Here's how the part is built. I have some questions about the finished solid (model axes, mm). Face numbers are marked on the shaded views. Give positions to 0.01 mm unless a question says otherwise; leave off trailing zeros. Write each loop counter-clockwise with the first axis right and the second up, starting at its lowest first coordinate (ties: lowest second). Pieces come first, ordered by that corner, then holes. Notation, with made-up numbers: (31, 26) -> (54, 26) arc R30 cw to (54, 50) -> close; hole circle Ø2 at (3.5, -25). An arc over 180 degrees is marked (long way). Put each result on its own line as item: value. Start each with the question number.
from build123d import *

# Parameters (mm, degrees)
SKETCH1_R             = 0.25
BOSS_EXTRUDE1_DEPTH   = 2.7
BOSS_EXTRUDE1_2_DEPTH = 2.7
BOSS_EXTRUDE1_3_DEPTH = 2.7
BOSS_EXTRUDE1_4_DEPTH = 2.7
BOSS_EXTRUDE1_5_DEPTH = 2.7
BOSS_EXTRUDE1_6_DEPTH = 2.7
BOSS_EXTRUDE1_7_DEPTH = 2.7
BOSS_EXTRUDE1_8_DEPTH = 2.7
SKETCH1_7_W           = 13.5
SKETCH1_7_H           = 2.85
SKETCH1_7_W_2         = 13.1
SKETCH1_7_H_2         = 2.45
BOSS_EXTRUDE3_DEPTH   = 2.7
SKETCH1_8_W           = 13.1
SKETCH1_8_H           = 2.45
SKETCH1_8_R           = 0.25
BOSS_EXTRUDE4_DEPTH   = 0.2
SKETCH1_9_R           = 0.25
BOSS_EXTRUDE5_DEPTH   = 2.7


with BuildPart() as part:
    # Sketch1 → Boss-Extrude1 (new body)
    with BuildSketch(Plane(origin=(0, 0, 0), x_dir=(1, 0, 0), z_dir=(0, 1, 0))):
        with Locations((-3.403301887, 0.02370283)):
            Circle(SKETCH1_R)
    extrude(amount=-BOSS_EXTRUDE1_DEPTH)



with BuildPart() as body_2:
    # Sketch1 → Boss-Extrude1 2 (new body)
    with BuildSketch(Plane(origin=(0, 0, 0), x_dir=(1, 0, 0), z_dir=(0, 1, 0))):
        with Locations((-1.903301887, 0.02370283)):
            Circle(SKETCH1_R)
    extrude(amount=-BOSS_EXTRUDE1_2_DEPTH)


with BuildPart() as body_3:
    # Sketch1 → Boss-Extrude1 3 (new body)
    with BuildSketch(Plane(origin=(0, 0, 0), x_dir=(1, 0, 0), z_dir=(0, 1, 0))):
        with Locations((-0.403301887, 0.02370283)):
            Circle(SKETCH1_R)
    extrude(amount=-BOSS_EXTRUDE1_3_DEPTH)


with BuildPart() as body_4:
    # Sketch1 → Boss-Extrude1 4 (new body)
    with BuildSketch(Plane(origin=(0, 0, 0), x_dir=(1, 0, 0), z_dir=(0, 1, 0))):
        with Locations((1.096698113, 0.02370283)):
            Circle(SKETCH1_R)
    extrude(amount=-BOSS_EXTRUDE1_4_DEPTH)


with BuildPart() as body_5:
    # Sketch1 → Boss-Extrude1 5 (new body)
    with BuildSketch(Plane(origin=(0, 0, 0), x_dir=(1, 0, 0), z_dir=(0, 1, 0))):
        with Locations((2.596698113, 0.02370283)):
            Circle(SKETCH1_R)
    extrude(amount=-BOSS_EXTRUDE1_5_DEPTH)


with BuildPart() as body_6:
    # Sketch1 → Boss-Extrude1 6 (new body)
    with BuildSketch(Plane(origin=(0, 0, 0), x_dir=(1, 0, 0), z_dir=(0, 1, 0))):
        with Locations((4.096698113, 0.02370283)):
            Circle(SKETCH1_R)
    extrude(amount=-BOSS_EXTRUDE1_6_DEPTH)


with BuildPart() as body_7:
    # Sketch1 → Boss-Extrude1 7 (new body)
    with BuildSketch(Plane(origin=(0, 0, 0), x_dir=(1, 0, 0), z_dir=(0, 1, 0))):
        with Locations((5.596698113, 0.02370283)):
            Circle(SKETCH1_R)
    extrude(amount=-BOSS_EXTRUDE1_7_DEPTH)


with BuildPart() as body_8:
    # Sketch1 → Boss-Extrude1 8 (new body)
    with BuildSketch(Plane(origin=(0, 0, 0), x_dir=(1, 0, 0), z_dir=(0, 1, 0))):
        with Locations((7.096698113, 0.02370283)):
            Circle(SKETCH1_R)
    extrude(amount=-BOSS_EXTRUDE1_8_DEPTH)


with BuildPart() as body_9:
    # Sketch1_7 → Boss-Extrude3 (new body)
    with BuildSketch(Plane(origin=(0, 0, 0), x_dir=(1, 0, 0), z_dir=(0, 1, 0))):
        with Locations((1.846698113, -0.098128497)):
            Rectangle(SKETCH1_7_W, SKETCH1_7_H)
        with Locations((1.846698113, -0.098128497)):
            Rectangle(SKETCH1_7_W_2, SKETCH1_7_H_2, mode=Mode.SUBTRACT)
    extrude(amount=BOSS_EXTRUDE3_DEPTH)

    # Sketch1_8 → Boss-Extrude4 (add)
    with BuildSketch(Plane(origin=(0, 0, 0), x_dir=(1, 0, 0), z_dir=(0, 1, 0))):
        with Locations((1.846698113, -0.098128497)):
            Rectangle(SKETCH1_8_W, SKETCH1_8_H)
        with Locations((-3.403301887, 0.02370283)):
            Circle(SKETCH1_8_R, mode=Mode.SUBTRACT)
        with Locations((-1.903301887, 0.02370283)):
            Circle(SKETCH1_8_R, mode=Mode.SUBTRACT)
        with Locations((-0.403301887, 0.02370283)):
            Circle(SKETCH1_8_R, mode=Mode.SUBTRACT)
        with Locations((1.096698113, 0.02370283)):
            Circle(SKETCH1_8_R, mode=Mode.SUBTRACT)
        with Locations((2.596698113, 0.02370283)):
            Circle(SKETCH1_8_R, mode=Mode.SUBTRACT)
        with Locations((4.096698113, 0.02370283)):
            Circle(SKETCH1_8_R, mode=Mode.SUBTRACT)
        with Locations((5.596698113, 0.02370283)):
            Circle(SKETCH1_8_R, mode=Mode.SUBTRACT)
        with Locations((7.096698113, 0.02370283)):
            Circle(SKETCH1_8_R, mode=Mode.SUBTRACT)
    extrude(amount=BOSS_EXTRUDE4_DEPTH)


with BuildPart() as part_1:
    add(part.part)

    add(body_2.part)  # Boss-Extrude5 merges body 2

    add(body_3.part)  # Boss-Extrude5 merges body 3

    add(body_4.part)  # Boss-Extrude5 merges body 4

    add(body_5.part)  # Boss-Extrude5 merges body 5

    add(body_6.part)  # Boss-Extrude5 merges body 6

    add(body_7.part)  # Boss-Extrude5 merges body 7

    add(body_8.part)  # Boss-Extrude5 merges body 8

    add(body_9.part)  # Boss-Extrude5 merges body 9
    # Sketch1_9 → Boss-Extrude5 (add)
    with BuildSketch(Plane(origin=(0, 0, 0), x_dir=(1, 0, 0), z_dir=(0, 1, 0))):
        with Locations((-3.403301887, 0.02370283)):
            Circle(SKETCH1_9_R)
        with Locations((-0.403301887, 0.02370283)):
            Circle(SKETCH1_9_R)
        with Locations((1.096698113, 0.02370283)):
            Circle(SKETCH1_9_R)
        with Locations((2.596698113, 0.02370283)):
            Circle(SKETCH1_9_R)
        with Locations((4.096698113, 0.02370283)):
            Circle(SKETCH1_9_R)
        with Locations((5.596698113, 0.02370283)):
            Circle(SKETCH1_9_R)
        with Locations((7.096698113, 0.02370283)):
            Circle(SKETCH1_9_R)
        with Locations((-1.903301887, 0.02370283)):
            Circle(SKETCH1_9_R)
    extrude(amount=BOSS_EXTRUDE5_DEPTH)


solid = part_1.part
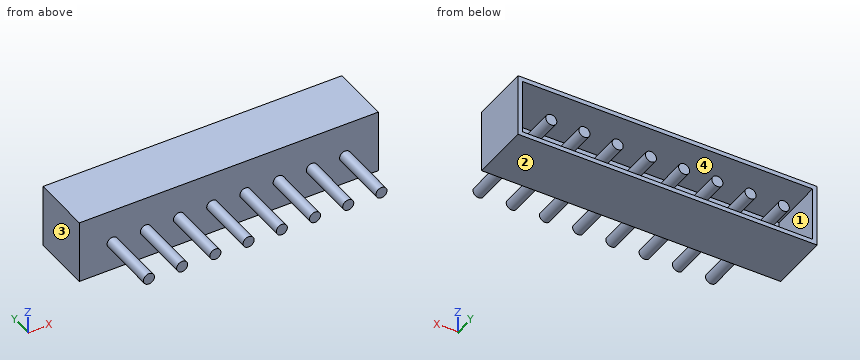
1) I want a section at A-A, the plane y = 2.05. State how many separate pieces and enclosed holes the cut face has, and give its area (3 significant figures).
2) I want a section at C-C, the plane x = -1. Write out the boundary of the cut face in (y, z).
3) I'm going to push flat-ended pins straight in: pin 1 Ø0.9 at (x, z) = (-1, -0.5) entering from -Y; pin 2 Ø1.2 at (x, z) = (3, 0) entering from +Y. Where does each tip first touch, or does it pass through?
4) I want a section at D-D, the plane y = -1.95. Write out the boundary of the cut face in (x, z), and give its area (3 significant figures).
5) I want a section at B-B, the plane z = 0.4. Write out the boundary of the cut face in (x, y), and give its area (3 significant figures).
6) Thinking about a two-plate mould opening in Z: for the marked faces 1, 2, 3 and 4, which applies, released by +Z, released by -Z, zero draft, split by the parting line, or undercut?
7) I need wall thicknesses on probe 1 along Z at (x, y) = (7.75, 0.7); probe 2 along Z at (x, y) = (-3.25, 1.8); probe 3 along Z at (x, y) = (-0.5, 2.15). Which ranges of each line are inside material? Lowest first, please.
Established:
1. separate pieces: 9
1. enclosed holes: 1
1. area: 7.95 mm2
2. outline: (0, -1.33) -> (2.7, -1.33) -> (2.7, -1.13) -> (0.2, -1.13) -> (0.2, 1.32) -> (2.7, 1.32) -> (2.7, 1.52) -> (0, 1.52) -> close
3. pin 1: stops at y = 0
3. pin 2: stops at y = 2.7
4. outline: circle Ø0.5 at (-3.4, -0.02); circle Ø0.5 at (-1.9, -0.02); circle Ø0.5 at (-0.4, -0.02); circle Ø0.5 at (1.1, -0.02); circle Ø0.5 at (2.6, -0.02); circle Ø0.5 at (4.1, -0.02); circle Ø0.5 at (5.6, -0.02); circle Ø0.5 at (7.1, -0.02)
4. area: 1.57 mm2
5. outline: (-4.9, 0) -> (8.6, 0) -> (8.6, 2.7) -> (8.4, 2.7) -> (8.4, 0.2) -> (-4.7, 0.2) -> (-4.7, 2.7) -> (-4.9, 2.7) -> close
5. area: 3.70 mm2
6. face 1: undercut
6. face 2: released by -Z
6. face 3: zero draft
6. face 4: undercut
7. probe 1: z = -1.33 to -1.13, 1.32 to 1.52
7. probe 2: z = -1.33 to -1.13, -0.22 to 0.17, 1.32 to 1.52
7. probe 3: z = -1.33 to -1.13, -0.25 to 0.21, 1.32 to 1.52
